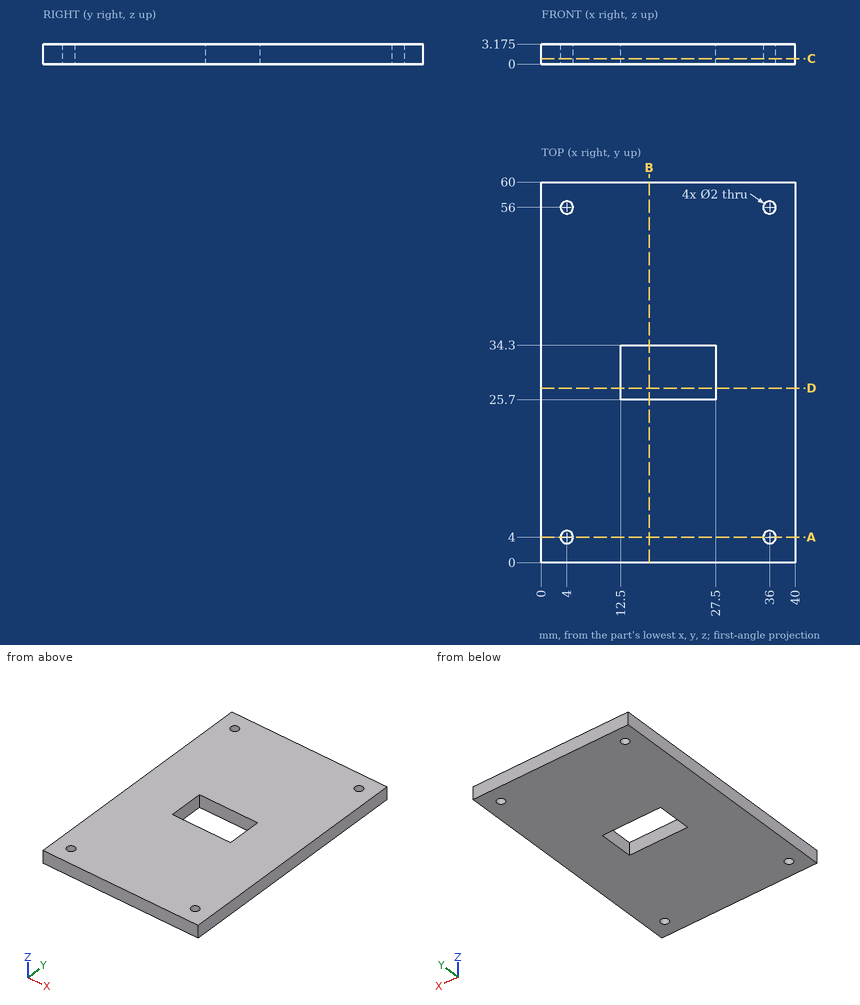
Drawing for the job (mm, zero at the part's lowest x, y, z). Coordinates: 2 decimals unless noted, no trailing zeros. Write each loop counter-clockwise with the first axis right and the second up, starting at its lowest first coordinate (ties: lowest second). Pieces come first, ordered by that corner, then holes. Notation, with made-up numbers: (29.25, 20) -> (47.25, 20) arc R6 cw to (47.25, 26) -> close; hole circle Ø10 at (-17.75, 56). An arc over 180 degrees is marked (long way). One line per item, written item: value. Start each with the question number.
1) Slice it at C-C on z = 0.85. Write the cut outline in (x, y).
2) Slice it at D-D on y = 27.5. Write the cut outline in (x, z) (3 decimals), then the cut area to 3 significant figures.
3) Slice it at B-B on x = 17. Write the cut outline in (y, z) (3 decimals), then the cut area to 3 significant figures.
4) Flat gauge pins, fed straight in: pin 1 Ø1.8 at (x, y) = (36, 4) entering from +Z; pin 2 Ø2.5 at (x, y) = (4, 4) entering from +Z (3 decimals). Where does each tip first touch, or does it go through?
5) Slice it at A-A on y = 4. Write the cut outline in (x, z) (3 decimals).
6) Probe probe 1 along Y at (x, z) = (4, 2.2); probe 2 along X at (y, z) = (28, 2.9); probe 3 along Y at (x, z) = (18, 0.7). List the from-to ranges inside material, lowest first.
Answers follow:
1. outline: (0, 0) -> (40, 0) -> (40, 60) -> (0, 60) -> close; hole circle Ø2 at (4, 4); hole circle Ø2 at (4, 56); hole (12.5, 25.7) -> (27.5, 25.7) -> (27.5, 34.3) -> (12.5, 34.3) -> close; hole circle Ø2 at (36, 4); hole circle Ø2 at (36, 56)
2. outline: (0, 0) -> (12.5, 0) -> (12.5, 3.175) -> (0, 3.175) -> close; (27.5, 0) -> (40, 0) -> (40, 3.175) -> (27.5, 3.175) -> close
2. area: 79.4 mm2
3. outline: (0, 0) -> (25.7, 0) -> (25.7, 3.175) -> (0, 3.175) -> close; (34.3, 0) -> (60, 0) -> (60, 3.175) -> (34.3, 3.175) -> close
3. area: 163 mm2
4. pin 1: through
4. pin 2: z = 3.175
5. outline: (0, 0) -> (3, 0) -> (3, 3.175) -> (0, 3.175) -> close; (5, 0) -> (35, 0) -> (35, 3.175) -> (5, 3.175) -> close; (37, 0) -> (40, 0) -> (40, 3.175) -> (37, 3.175) -> close
6. probe 1: 0 to 3, 5 to 55, 57 to 60
6. probe 2: 0 to 12.5, 27.5 to 40
6. probe 3: 0 to 25.7, 34.3 to 60
